Geometry: see drawing. Coordinates: mm, zero at the bounding-box minimum. A direction names the side the tool comes from. Give positions to 0.01 mm unless a question says otherwise; leave off trailing zeros. Order: outer loops, then holes, each group sorted by start corner. A loop starts at its lowest first (then second) coordinate and runs counter-clockwise, first axis right, second up. Notation, with made-up numbers: (-37, 17.5) - (12, 17.5) arc R4 ccw to (12, 23.5) - close; hole circle Ø1 at (49.5, 79.5). An arc over 180 degrees is marked (long way). Write item = value, one per line. Start each with the question number.
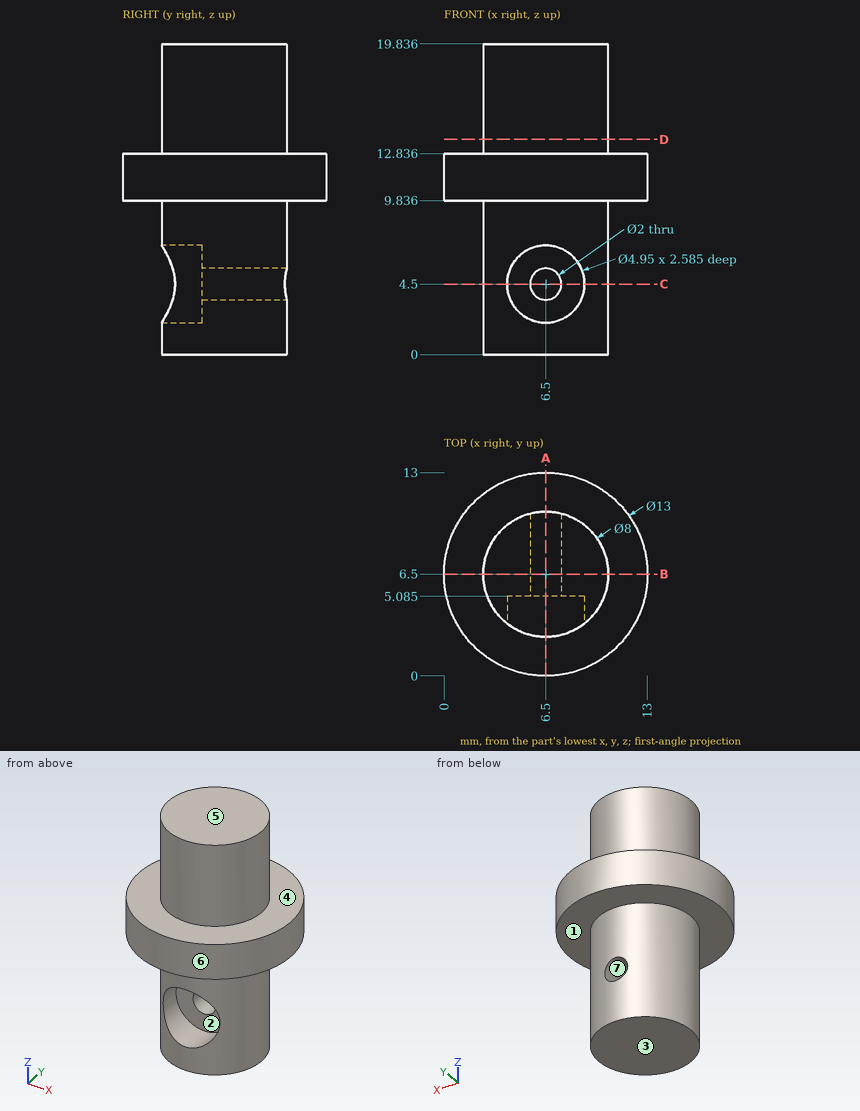
Q1. Contact query for flat-ended pins moving along their axis: pin 1 (3 mm diameter, centred on x = 6.5, z = 4.5, fed in from -Y) (3 decimals); pin 2 (5 mm diameter, centred on x = 9.5, z = 4, fed in from -Y); pin 3 (4 mm diameter, centred on x = 3.5, z = 15.5, fed in from -Y). Output: stop coordinate, or through.
Q2. Section C-C, the plane z = 4.5. Return the cut outline in (x, y) (1 decimal).
Q3. Set-up query: the marked faces 1, 2, 3 and 4. Return all of +Z, -Z, +X, -X, +Y, -Y with unobstructed straight access to the full face (end or side cutting, diameter ignored); none if empty.
Q4. Section D-D, the plane z = 13.75. Return the cut outline in (x, y), then the cut area to 3 significant figures.
Q5. Section B-B, the plane y = 6.5. Return the cut outline in (x, z), then the cut area to 3 significant figures.
Q6. Pull-direction query (Z, two-part tool) for the marked faces 5, 6 and 7; classes: +Z half, -Z half, draft (parallel to the pull), parting line (faces both ways), or undercut.
Q7. Material intervals for line 1 along Z through (x, y) = (6.5, 3.35) (1 decimal); line 2 along Z through (x, y) = (6.5, 7.1); line 3 along Z through (x, y) = (10.75, 2.25), sorted ascending. Write a range as from..to.
Q8. Section A-A, the plane x = 6.5. Return the cut outline in (y, z) (1 decimal), then the cut area to 3 significant figures.
The answers:
q1.pin_1 = 5.085
q1.pin_2 = 2.67
q1.pin_3 = 2.63
q2.outline = (4, 3.4) - (4, 5.1) - (5.5, 5.1) - (5.5, 10.4) arc R4 ccw to start; (7.5, 5.1) - (9, 5.1) - (9, 3.4) arc R4 ccw to (7.5, 10.4) - close
q3.face_1 = -Z
q3.face_2 = -Y
q3.face_3 = -Z, +X, -X, +Y, -Y
q3.face_4 = +Z
q4.outline = circle Ø8 at (6.5, 6.5)
q4.area = 50.3 mm²
q5.outline = (0, 9.84) - (2.5, 9.84) - (2.5, 0) - (10.5, 0) - (10.5, 9.84) - (13, 9.84) - (13, 12.84) - (10.5, 12.84) - (10.5, 19.84) - (2.5, 19.84) - (2.5, 12.84) - (0, 12.84) - close; hole circle Ø2 at (6.5, 4.5)
q5.area = 171 mm²
q6.face_5 = +Z half
q6.face_6 = draft
q6.face_7 = undercut
q7.line_1 = 0..2, 7..19.8
q7.line_2 = 0..3.5, 5.5..19.84
q7.line_3 = 9.84..12.84
q8.outline = (0, 9.8) - (2.5, 9.8) - (2.5, 7) - (5.1, 7) - (5.1, 5.5) - (10.5, 5.5) - (10.5, 9.8) - (13, 9.8) - (13, 12.8) - (10.5, 12.8) - (10.5, 19.8) - (2.5, 19.8) - (2.5, 12.8) - (0, 12.8) - close; (2.5, 0) - (10.5, 0) - (10.5, 3.5) - (5.1, 3.5) - (5.1, 2) - (2.5, 2) - close
q8.area = 150 mm²
